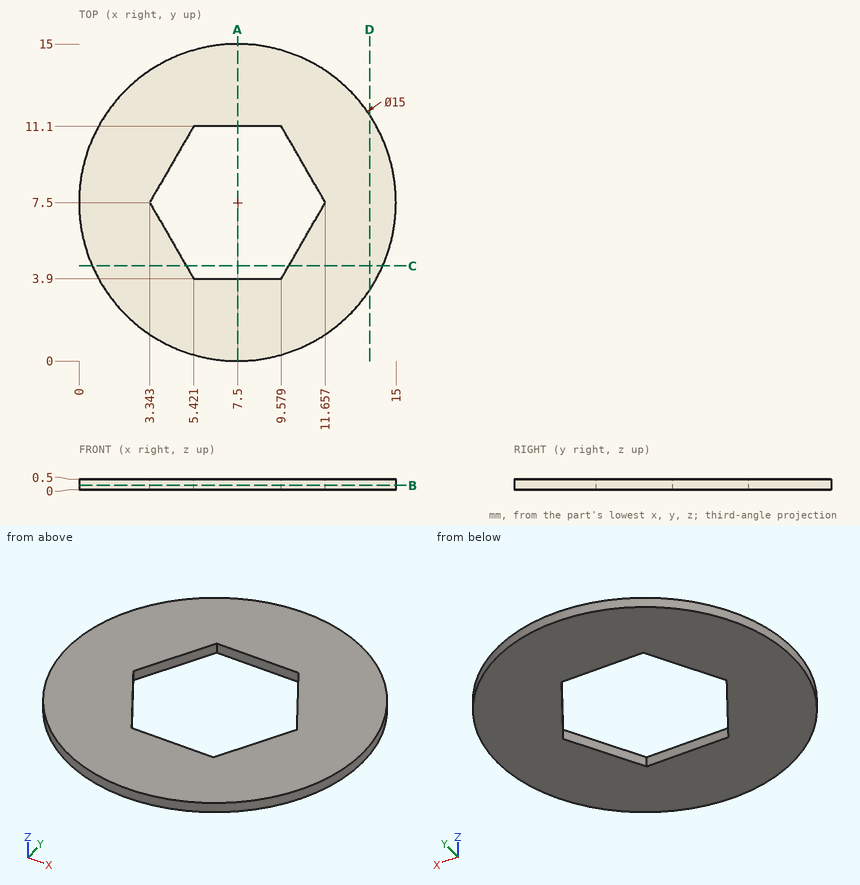
Verification items for this drawing (mm, ordinates from the low corner). Coordinates: 2 decimals unless noted, no trailing zeros. Loops run counter-clockwise (first coordinate to the right, second up) from the corner with the lowest first, then second, coordinate; pieces in that order, holes last.
Item 1: Thickness scan on line 1 (X direction, y = 5.5, z = 0.1); line 2 (X direction, y = 11, z = 0.1) (1 decimal); line 3 (Y direction, x = 4.75, z = 0.25) (1 decimal). Record the ranges inside material, lowest first.
Item 2: Sectioned sample at C-C, the plane y = 4.5. Record the boundary of the cut face in (x, z) (1 decimal).
Item 3: Sectioned sample at B-B, the plane z = 0.2. Record the boundary of the cut face in (x, y), then the cut area to 3 significant figures.
Item 4: Sectioned sample at A-A, the plane x = 7.5. Record the boundary of the cut face in (y, z).
Item 5: Sectioned sample at D-D, the plane x = 13.75. Record the boundary of the cut face in (y, z) (1 decimal).
Check result:
1. line 1: x = 0.27 to 4.5, 10.5 to 14.73
1. line 2: x = 0.9 to 5.4, 9.6 to 14.1
1. line 3: y = 0.5 to 5.1, 9.9 to 14.5
2. outline: (0.6, 0) - (5.1, 0) - (5.1, 0.5) - (0.6, 0.5) - close; (9.9, 0) - (14.4, 0) - (14.4, 0.5) - (9.9, 0.5) - close
3. outline: circle Ø15 at (7.5, 7.5); hole (3.34, 7.5) - (5.42, 3.9) - (9.58, 3.9) - (11.66, 7.5) - (9.58, 11.1) - (5.42, 11.1) - close
3. area: 132 mm2
4. outline: (0, 0) - (3.9, 0) - (3.9, 0.5) - (0, 0.5) - close; (11.1, 0) - (15, 0) - (15, 0.5) - (11.1, 0.5) - close
5. outline: (3.4, 0) - (11.6, 0) - (11.6, 0.5) - (3.4, 0.5) - close
